Verification items for the finished model (mm, model axes). Give positions to 0.01 mm unless a question says otherwise; leave off trailing zeros. Loops run counter-clockwise (first coordinate to the right, second up) from the corner with the lowest first, then second, coordinate; pieces in that order, holes last. Notation, with made-up numbers: (-0.75, 0.25) -> (23.25, 0.25) arc R25 ccw to (23.25, 33.25) -> close; hole circle Ø2 at (14, 85). An arc over 180 degrees is marked (long way). Answer in a Markdown table with one row per item. Add a question column.
Q1. Section check A-A on y = 0. Enter the section's corners in (x, z), and give its area (3 significant figures).
Q2. Gauge pin test, flat ends, axial feed: P1, Ø8, axis at x = 45, y = -31.5, coming from the -Z side; P2, Ø12, axis at x = 40.5, y = 21, coming from the +Z side; P3, Ø12, axis at x = 10.5, z = -17, coming from the -Y side. Record the tip position at first contact, or that the pin passes through.
Q3. Section check C-C on x = 28. Enter the section's corners in (y, z).
Q4. Section check D-D on x = 7. Enter the section's corners in (y, z), and give its area (3 significant figures).
Q5. Material ranges on probe 1 along Z at (x, y) = (31, 0); probe 2 along Z at (x, y) = (56.5, -1), recorded low to high.
Q6. Release check for a two-part mould opening along X. For faces 1 (the face through (39.25, -37.66, -28.88)), 2 (the face through (39.25, 47.69, 15.02)) record: pulls with the +X half, pulls with the -X half, needs draft (parallel to the pull), parting line crosses it, or undercut.
```python
from build123d import *

# Parameters (mm, degrees)
F0_R     = 50
F1_DEPTH = 78.994
F2_R     = 22.0755688143
F3_T     = -2.54


# Not quite as in the source:
# - a fillet or chamfer that OpenCascade refuses, or shapes differently, is made with other operations: its cross-section is extruded or revolved along the edge and cut away or added


with BuildPart() as f1:
    # F0 (on Right) → F1 (new body)
    with BuildSketch(Plane.YZ):
        Circle(F0_R)
    extrude(amount=F1_DEPTH)

    # F2
    f2_edges = [f1.edges().sort_by_distance(p)[0] for p in [
        (78.994, -50, 0),
        (0, -50, 0),
        (39.497, 50, 0),
    ]]
    fillet(f2_edges, radius=F2_R)

    # F3: a shell. OpenCascade refuses it in one call, so the cavity is built on its own and cut out:
    # the body offset inwards by the wall thickness, plus a prism from it out through each open face.
    f3_core = offset(f1.part, amount=F3_T, mode=Mode.PRIVATE)
    f3_exits = [f3_core.faces().sort_by_distance(p)[0] for p in [
        (76.454, 0, 0),
        (2.54, 0, 0),
    ]]
    add(f3_core, mode=Mode.SUBTRACT)
    extrude(f3_exits, amount=-F3_T, mode=Mode.SUBTRACT)

    # F4: fillet of radius 5.08 on 6 edges, made by hand

    # F4_s1 → F4_t2 (revolve, cut)
    with BuildSketch(Plane.XY):
        with BuildLine():
            ThreePointArc((0.6434411467, 33.2154275111), (0.793307898, 30.2837381407), (2.54, 27.9244311857))
            Line((2.54, 27.9244311857), (0, 27.9244311857))
            ThreePointArc((0, 27.9244311857), (0.1614506751, 30.5894198641), (0.6434411467, 33.2154275111))
        make_face()
    revolve(axis=Axis((0, 0, 0), (1, 0, 0)), mode=Mode.SUBTRACT)

    # F4_s3 → F4_t4 (revolve, cut)
    with BuildSketch(Plane.XY):
        with BuildLine():
            ThreePointArc((78.3505588533, 33.2154275111), (78.200692102, 30.2837381407), (76.454, 27.9244311857))
            Line((76.454, 27.9244311857), (78.994, 27.9244311857))
            ThreePointArc((78.994, 27.9244311857), (78.8325493249, 30.5894198641), (78.3505588533, 33.2154275111))
        make_face()
    revolve(axis=Axis((78.994, 0, 0), (1, 0, 0)), mode=Mode.SUBTRACT)


solid = f1.part
```
Taken from the geometry:
| question | item | result |
|---|---|---|
| 1 | outline | (0.64, -33.22) arc R22.08 ccw to (22.08, -50) -> (56.92, -50) arc R22.08 ccw to (78.35, -33.22) arc R5.08 ccw to (76.45, -27.92) arc R19.54 cw to (56.92, -47.46) -> (22.08, -47.46) arc R19.54 cw to (2.54, -27.92) arc R5.08 ccw to start; (0.64, 33.22) arc R5.08 ccw to (2.54, 27.92) arc R19.54 cw to (22.08, 47.46) -> (56.92, 47.46) arc R19.54 cw to (76.45, 27.92) arc R5.08 ccw to (78.35, 33.22) arc R22.08 ccw to (56.92, 50) -> (22.08, 50) arc R22.08 ccw to start |
| 1 | area | 493 mm² |
| 2 | P1 | stops at z = -41.76 |
| 2 | P2 | stops at z = 47.7 |
| 2 | P3 | stops at y = -47.07 |
| 3 | outline | circle Ø100 at (0, 0); hole circle Ø94.92 at (0, 0) |
| 4 | outline | circle Ø88.1 at (0, 0); hole circle Ø80.7 at (0, 0) |
| 4 | area | 982 mm² |
| 5 | probe 1 | z = -50 to -47.46, 47.46 to 50 |
| 5 | probe 2 | z = -49.99 to -47.45, 47.45 to 49.99 |
| 6 | face 1 | undercut |
| 6 | face 2 | needs draft |
